Job drawing, mm, ordinate dimensions from the low corner. One solid piece. A direction names the side the tool comes from. Round coordinates to 2 decimals unless told otherwise and drop trailing zeros. Loops run counter-clockwise (first coordinate to the right, second up) from the corner with the lowest first, then second, coordinate; pieces in that order, holes last.
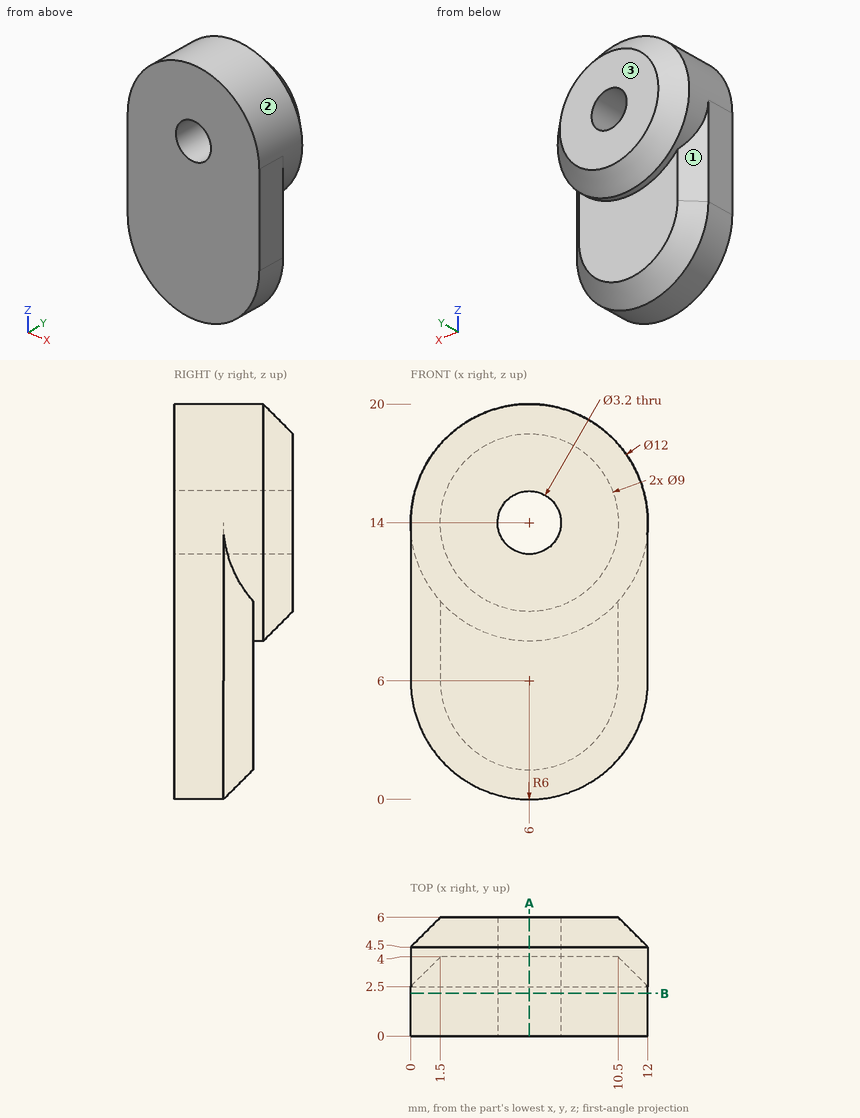
(1) Probe line 1 (X direction, y = 4.35, z = 14); line 2 (Y direction, x = 10, z = 6); line 3 (Z direction, x = 5.75, y = 1.35). List the from-to ranges inside material, lowest first.
Responses:
line 1: x = 0 to 4.4, 7.6 to 12
line 2: y = 0 to 4
line 3: z = 0.01 to 12.42, 15.58 to 19.99
(2) Slice it at A-A on x = 6. List the corners of the cut face in (y, z), plus the area to 3 significant figures.
Responses:
outline: (0, 0) - (2.5, 0) - (4, 1.5) - (4, 8) - (4.5, 8) - (6, 9.5) - (6, 12.4) - (0, 12.4) - close; (0, 15.6) - (6, 15.6) - (6, 18.5) - (4.5, 20) - (0, 20) - close
area: 81.4 mm2
(3) Slice it at B-B on y = 2.15. List the corners of the cut face in (x, z), plus the area to 3 significant figures.
Responses:
outline: (0, 6) arc R6 ccw to (12, 6) - (12, 14) arc R6 ccw to (0, 14) - close; hole circle Ø3.2 at (6, 14)
area: 201 mm2
(4) Which spindle directions (+Z, -Z, +X, -X, +Y, -Y) get a long thin tool onto all of the face, cutting with end or side? Do the marked faces 1, 2 and 3. Say none if no direction does.
Responses:
face 1: -Z, -X, +Y
face 2: +Y
face 3: +Z, -Z, +X, -X, +Y
